Input: dimensioned drawing with shaded views. Units: mm. Origin: part minimum x, y, z. A direction names the side the tool comes from. Give positions to 0.01 mm unless a question says otherwise; leave off trailing zeros. Loops run counter-clockwise (first coordinate to the right, second up) from the corner with the lowest first, then second, coordinate; pieces in that order, holes last. Notation, with made-up numbers: (15, 89.25) -> (23, 89.25) arc R20 ccw to (23, 108.25) -> close; hole circle Ø1 at (3.5, 58). An arc over 180 degrees is marked (long way). Answer as a JSON object with one key per item and string values.
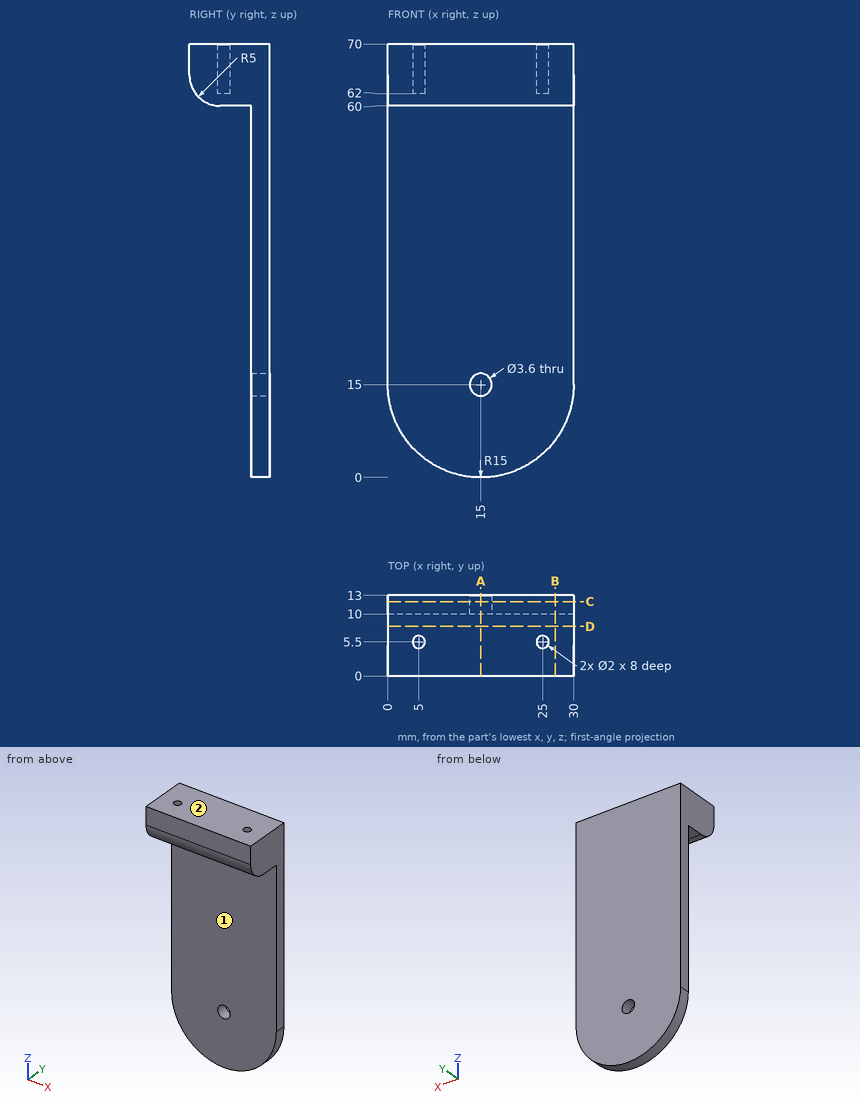
Q1. Pin query (flat end, axial travel): pin 1 (1 mm diameter, centred on x = 8.5, y = 8, fed in from -Z); pin 2 (15 mm diameter, centred on x = 21, z = 41.5, fed in from -Y); pin 3 (0.6 mm diameter, centred on x = 25, y = 5.5, fed in from +Z); pin 4 (1 mm diameter, centred on y = 9, z = 46, fed in from +X). Return the tip coordinate at first contact, or that it passes through.
Evaluation:
{"pin 1": "stops at z = 60", "pin 2": "stops at y = 10", "pin 3": "stops at z = 62", "pin 4": "passes through"}
Q2. Section C-C, the plane y = 12. Return the cut outline in (x, z).
Evaluation:
{"outline": "(0, 15) arc R15 ccw to (30, 15) -> (30, 70) -> (0, 70) -> close; hole circle Ø3.6 at (15, 15)"}
Q3. Section D-D, the plane y = 8. Return the cut outline in (x, z).
Evaluation:
{"outline": "(0, 60) -> (30, 60) -> (30, 70) -> (0, 70) -> close"}
Q4. Section B-B, the plane x = 27. Return the cut outline in (y, z).
Evaluation:
{"outline": "(0, 65) arc R5 ccw to (5, 60) -> (10, 60) -> (10, 6) -> (13, 6) -> (13, 70) -> (0, 70) -> close"}
Q5. Access query for the marked faces 1 and 2. Directions: +Z, -Z, +X, -X, +Y, -Y. A direction counts if a zero-diameter tool reaches every point of the face in a straight line with its end or side. Return the directions, or none.
Evaluation:
{"face 1": "-Z, +X, -X, -Y", "face 2": "+Z, +X, -X, +Y, -Y"}
Q6. Section A-A, the plane x = 15. Return the cut outline in (y, z), then the cut area to 3 significant figures.
Evaluation:
{"outline": "(0, 65) arc R5 ccw to (5, 60) -> (10, 60) -> (10, 16.8) -> (13, 16.8) -> (13, 70) -> (0, 70) -> close; (10, 0) -> (13, 0) -> (13, 13.2) -> (10, 13.2) -> close", "area": "294 mm2"}
Q7. Ray query, line 1 along Y through (x, z) = (5, 65); line 2 along X through (y, z) = (11.5, 15); line 3 along Y through (x, z) = (2, 12). Return the intervals inside material, ascending.
Evaluation:
{"line 1": "y = 0 to 4.5, 6.5 to 13", "line 2": "x = 0 to 13.2, 16.8 to 30", "line 3": "y = 10 to 13"}
